Here's how the part is built. I have some questions about the finished solid (model axes, mm). A direction names the side the tool comes from. Give positions to 0.01 mm unless a question says otherwise; leave off trailing zeros. Write each loop counter-clockwise with the first axis right and the second up, starting at its lowest first coordinate (ties: lowest second). Pieces come first, ordered by that corner, then holes. Notation, with made-up numbers: (-29, 68.5) -> (26, 68.5) arc R26 cw to (26, 86.5) -> close; hole circle Ø4 at (26.25, 13). An arc over 180 degrees is marked (long way). Return JSON: item names as keys, results as strings.
from build123d import *

# Parameters (mm, degrees)
F0_R     = 12.7
F1_DEPTH = 28.575
F2_R     = 6.7437
F3_DEPTH = 28.575
F5_R     = 4.7625
F6_DEPTH = 19.4447


with BuildPart() as f1:
    # F0 (on Top) → F1 (new body)
    with BuildSketch(Plane.XY):
        Circle(F0_R)
    extrude(amount=F1_DEPTH)

    # F2 (on face) → F3 (join)
    with BuildSketch(Plane.XY.offset(28.575)):
        Circle(F2_R)
    extrude(amount=F3_DEPTH)

    # F5 (on offset) → F6 (cut, through all)
    with BuildSketch(Plane.XZ.offset(6.7437)):
        with Locations((0, 42.8498)):
            Circle(F5_R)
    extrude(amount=-F6_DEPTH, mode=Mode.SUBTRACT)


solid = f1.part
1. For pin 1 Ø12 at (y, z) = (9.5, 40) entering from +X; pin 2 Ø4 at (x, z) = (6, 24) entering from +Y; pin 3 Ø4 at (x, y) = (7, 6) entering from -Z; pin 4 Ø8.5 at (x, z) = (0, 42.85) entering from +Y, each with a flat end and sliding along its axis, tell me the tip position at first contact or that it passes through.
Taken from the geometry:
{"pin 1": "stops at x = 5.76", "pin 2": "stops at y = 12.05", "pin 3": "stops at z = 0", "pin 4": "passes through"}
2. If we mould it in two halves opening along X, with no side actions, what happens to faces 3 (the face through (-2.75, -12.4, 14.09)), 4 (the face through (0, 0, 57.15)), 5 (the face through (4.543, -0.088, 44.28))? For each: released by +X, released by -X, zero draft, split by the parting line, or undercut.
Taken from the geometry:
{"face 3": "split by the parting line", "face 4": "zero draft", "face 5": "undercut"}
3. If I drill on line 1 (Z direction, x = 0, y = -3); line 2 (Z direction, x = 4.75, y = -8) (3 decimals); line 3 (Z direction, x = 1, y = -3.5), over which ranges is the centre line in solid material (lowest first)? Write a range as [from, to].
Taken from the geometry:
{"line 1": "z = [0, 38.09], [47.61, 57.15]", "line 2": "z = [0, 28.575]", "line 3": "z = [0, 38.19], [47.51, 57.15]"}
4. Suppose I cut it at D-D, the plane z = 39. List the corners of the cut face in (x, y) for me.
Taken from the geometry:
{"outline": "(-2.8, -6.13) -> (-2.8, 6.13) arc R6.74 ccw to start; (2.8, -6.13) arc R6.74 ccw to (2.8, 6.13) -> close"}
5. Suppose I cut it at A-A, the plane x = 0. List the corners of the cut face in (y, z) for me (3 decimals).
Taken from the geometry:
{"outline": "(-12.7, 0) -> (12.7, 0) -> (12.7, 28.575) -> (6.744, 28.575) -> (6.744, 38.087) -> (-6.744, 38.087) -> (-6.744, 28.575) -> (-12.7, 28.575) -> close; (-6.744, 47.612) -> (6.744, 47.612) -> (6.744, 57.15) -> (-6.744, 57.15) -> close"}
6. Suppose I cut it at C-C, the plane z = 50. List the corners of the cut face in (x, y) for me, and give its area (3 significant figures).
Taken from the geometry:
{"outline": "circle Ø13.49 at (0, 0)", "area": "143 mm²"}
7. Which directions (+Z, -Z, +X, -X, +Y, -Y) give clear straight access to the entire face, cutting with the end or side of a thin tool? Please do faces 1 (the face through (0, 0, 0)), 2 (the face through (5, -5, 28.575)).
Taken from the geometry:
{"face 1": "-Z, +X, -X, +Y, -Y", "face 2": "+Z"}
